Here's how the part is built. I have some questions about the finished solid (model axes, mm). A direction names the side the tool comes from. Coordinates: 2 decimals unless noted, no trailing zeros. Order: outer loops, then holes, each group sorted by start corner. A loop starts at its lowest first (then second) coordinate and runs counter-clockwise, first axis right, second up. Notation, with made-up numbers: (18, 78) - (64, 78) arc R23 cw to (64, 105) - close; hole circle Ø4 at (-7.5, 39.5). An arc over 180 degrees is marked (long way). Use one line per item in the form item = value. Start each with the question number.
from build123d import *

# Parameters (mm, degrees)
SKETCH_1_W          = 33
SKETCH_1_H          = 27
EXTRUDE_1_DEPTH     = 5
FILLET_1_R          = 2
SKETCH_2_R          = 1
EXTRUDE_2_DEPTH     = 8
SKETCH_3_W          = 10
SKETCH_3_H          = 10
EXTRUDE_3_DEPTH     = 6
CHAMFER_1_SIZE      = 1
CUT_EXTRUDE_1_DEPTH = 4
SKETCH_5_W          = 14.5
SKETCH_5_H          = 9
SKETCH_5_W_2        = 2.4
SKETCH_5_H_2        = 7.7
EXTRUDE_4_DEPTH     = 11
SKETCH_6_R          = 2.85
SKETCH_6_R_2        = 0.5
CUT_EXTRUDE_2_DEPTH = 8
CUT_EXTRUDE_2_DRAFT = -3
CUT_EXTRUDE_3_DEPTH = 11
EXTRUDE_5_DEPTH     = 7.5
SKETCH_9_W          = 7
SKETCH_9_H          = 4
EXTRUDE_6_DEPTH     = 4.3
FILLET_2_R          = 1
CUT_EXTRUDE_START   = -3.5
SKETCH_10_R         = 1.5
CUT_EXTRUDE_4_DEPTH = 2.5


with BuildPart() as part:
    # 草图1 → 凸台-拉伸1 (new body)
    with BuildSketch(Plane.XY):
        with Locations((16.5, 13.5)):
            Rectangle(SKETCH_1_W, SKETCH_1_H)
    extrude(amount=EXTRUDE_1_DEPTH)

    # 圆角1
    fillet_1_edges = [part.edges().sort_by_distance(p)[0] for p in [
        (33, 27, 2.5),
        (33, 0, 2.5),
    ]]
    fillet(fillet_1_edges, radius=FILLET_1_R)

    # 草图2 → 凸台-拉伸2 (add)
    with BuildSketch(Plane(origin=(0, 0, 0), x_dir=(-1, 0, 0), z_dir=(0, 0, -1))):
        with Locations((-17.2, 23.2)):
            Circle(SKETCH_2_R)
        with Locations((-29.5, 23.2)):
            Circle(SKETCH_2_R)
        with Locations((-29.5, 3.8)):
            Circle(SKETCH_2_R)
        with Locations((-17.2, 3.8)):
            Circle(SKETCH_2_R)
    extrude(amount=EXTRUDE_2_DEPTH)

    # 草图3 → 凸台-拉伸3 (add)
    with BuildSketch(Plane.XY.offset(5)):
        with Locations((28, 13.5)):
            Rectangle(SKETCH_3_W, SKETCH_3_H)
    extrude(amount=EXTRUDE_3_DEPTH)

    # 倒角1
    chamfer_1_edges = [part.edges().sort_by_distance(p)[0] for p in [
        (23, 8.5, 8),
    ]]
    chamfer(chamfer_1_edges, length=CHAMFER_1_SIZE)

    # 草图4 → 切除-拉伸1 (cut)
    with BuildSketch(Plane.XY.offset(11)):
        Polygon((24, 17.5), (27, 17.5), (27, 9.5), (25, 9.5), (24, 10.5), align=None)
        Polygon((29, 17.5), (32, 17.5), (32, 9.5), (30, 9.5), (29, 10.5), align=None)
    extrude(amount=-CUT_EXTRUDE_1_DEPTH, mode=Mode.SUBTRACT)

    # 草图5 → 凸台-拉伸4 (add)
    with BuildSketch(Plane.XY.offset(5)):
        with Locations((7.25, 20.5)):
            Rectangle(SKETCH_5_W, SKETCH_5_H)
        with Locations((9.8, 4.35)):
            Rectangle(SKETCH_5_W_2, SKETCH_5_H_2)
    extrude(amount=EXTRUDE_4_DEPTH)


with BuildPart() as cut_extrude_2_tool:
    # 草图6 → 切除-拉伸2 (with draft: the straight prism first)
    with BuildSketch(Plane.ZY):
        with Locations((11.55, 20.5)):
            Circle(SKETCH_6_R)
        with Locations((11.55, 20.5)):
            Circle(SKETCH_6_R_2, mode=Mode.SUBTRACT)
    extrude(amount=-CUT_EXTRUDE_2_DEPTH)
    # 切除-拉伸2: the draft: its side faces are tilted about the plane it starts from
    cut_extrude_2_sides = [cut_extrude_2_tool.faces().sort_by_distance(p)[0] for p in [
        (4, 20.5, 8.7),
        (4, 20.5, 11.05),
    ]]
    draft(cut_extrude_2_sides, Plane.ZY, CUT_EXTRUDE_2_DRAFT)


with BuildPart() as part_1:
    add(part.part)

    # 切除-拉伸2: cut by cut_extrude_2_tool
    add(cut_extrude_2_tool.part, mode=Mode.SUBTRACT)

    # 草图7 → 切除-拉伸3 (cut)
    with BuildSketch(Plane(origin=(14.5, 0, 0), x_dir=(0, 0, -1), z_dir=(1, 0, 0))):
        Polygon((-14.5, 18), (-14.5, 23), (-12.5, 25), (-16, 25), (-16, 16), (-12.5, 16), align=None)
    extrude(amount=-CUT_EXTRUDE_3_DEPTH, mode=Mode.SUBTRACT)

    # 草图8 → 凸台-拉伸5 (add)
    with BuildSketch(Plane.ZY):
        with BuildLine():
            Line((8.1, 9.95), (8.1, 4.15))
            ThreePointArc((8.1, 4.15), (6.55, 2.6), (5, 4.15))
            Line((5, 4.15), (5, 9.95))
            ThreePointArc((5, 9.95), (6.55, 11.5), (8.1, 9.95))
        make_face()
        with BuildLine():
            Line((7.6, 9.95), (7.6, 4.15))
            ThreePointArc((7.6, 4.15), (6.55, 3.1), (5.5, 4.15))
            Line((5.5, 4.15), (5.5, 9.95))
            ThreePointArc((5.5, 9.95), (6.55, 11), (7.6, 9.95))
        make_face(mode=Mode.SUBTRACT)
    extrude(amount=-EXTRUDE_5_DEPTH)

    # 草图9 → 凸台-拉伸6 (add)
    with BuildSketch(Plane.XY.offset(5)):
        with Locations((23, 24.5)):
            Rectangle(SKETCH_9_W, SKETCH_9_H)
        with Locations((23, 2.5)):
            Rectangle(SKETCH_9_W, SKETCH_9_H)
    extrude(amount=EXTRUDE_6_DEPTH)

    # 圆角2
    fillet_2_edges = [part_1.edges().sort_by_distance(p)[0] for p in [
        (1.75, 16, 16),
        (8.6, 4.35, 16),
        (9.8, 0.5, 16),
        (11, 4.35, 16),
        (9.8, 8.2, 16),
        (1.75, 25, 16),
        (0, 27, 2.5),
        (0, 0, 2.5),
    ]]
    fillet(fillet_2_edges, radius=FILLET_2_R)

    # 草图10 → 切除-拉伸4 (cut)
    with BuildSketch(Plane(origin=(0, 0, 0), x_dir=(-1, 0, 0), z_dir=(0, 0, -1)).offset(CUT_EXTRUDE_START)):
        with BuildLine():
            ThreePointArc((-33, 2), (-32.414213562, 0.585786438), (-31, 0))
            Line((-31, 0), (-1, 0))
            ThreePointArc((-1, 0), (-0.292893219, 0.292893219), (0, 1))
            Line((0, 1), (0, 26))
            ThreePointArc((0, 26), (-0.292893219, 26.707106781), (-1, 27))
            Line((-1, 27), (-31, 27))
            ThreePointArc((-31, 27), (-32.414213562, 26.414213562), (-33, 25))
            Line((-33, 25), (-33, 2))
        make_face()
        with Locations((-17.2, 3.8)):
            Circle(SKETCH_10_R, mode=Mode.SUBTRACT)
        with Locations((-29.5, 3.8)):
            Circle(SKETCH_10_R, mode=Mode.SUBTRACT)
        with Locations((-17.2, 23.2)):
            Circle(SKETCH_10_R, mode=Mode.SUBTRACT)
        with Locations((-29.5, 23.2)):
            Circle(SKETCH_10_R, mode=Mode.SUBTRACT)
    extrude(amount=CUT_EXTRUDE_4_DEPTH, mode=Mode.SUBTRACT)


solid = part_1.part
1) Suppose I cut it at C-C, the plane x = 4. List the corners of the cut face in (y, z) for me, then the cut area to 3 significant figures.
2) I need wall thicknesses on probe 1 along Y at (x, z) = (5, 6.5); probe 2 along Z at (x, y) = (25.5, 16.5); probe 3 along X at (y, z) = (17.5, 6). Which ranges of each line are inside material? Lowest first, please. Write a range as [from, to].
3) Suppose I cut it at A-A, the plane x = 23.5. List the corners of the cut face in (y, z) for me, then the cut area to 3 significant figures.
4) For pin 1 (2 mm diameter, centred on x = 7.5, y = 5.5, fed in from +Z); pin 2 (8 mm diameter, centred on x = 24.5, z = 12, fed in from -Y); pin 3 (5 mm diameter, centred on x = 30.5, z = 8.5, fed in from +Y), each with a flat end and sliding along its axis, tell me the tip position at first contact or that it passes through.
5) If we mould it in two halves opening along Y, with no side actions, what happens to faces 1 (the flat face through (0, 13.3, 0.5)), 2 (the cylindrical face through (32.4, 0.57, 4.26)), 3 (the cylindrical face through (30.61, 24.21, 2.27))? For each: pulls with the +Y half, pulls with the -Y half, needs draft (parallel to the pull), parting line crosses it, or undercut.
6) Suppose I cut it at B-B, the plane z = 11.55. List the corners of the cut face in (x, y) for me.
7) Which directions (+Z, -Z, +X, -X, +Y, -Y) give clear straight access to the entire face, cutting with the end or side of a thin tool? Please do faces 4 (the flat face through (10, 0.5, 10)), 5 (the flat face through (8.6, 4, 10)), 6 (the flat face through (9.1, 17, 13.5)), 7 (the flat face through (23, 25, 9.3)), 8 (the flat face through (23, 3, 9.3)).
From the geometry:
q1.outline = (0, 0) - (27, 0) - (27, 1) - (0, 1) - close; (0, 3.5) - (27, 3.5) - (27, 5) - (25, 5) - (25, 12.5) - (23, 14.5) - (18, 14.5) - (16, 12.5) - (16, 5) - (9.95, 5) arc R1.55 ccw to (9.95, 8.1) - (4.15, 8.1) arc R1.55 ccw to (4.15, 5) - (0, 5) - close; circle Ø1.42 at (20.5, 11.55); hole (4.15, 5.5) - (9.95, 5.5) arc R1.05 ccw to (9.95, 7.6) - (4.15, 7.6) arc R1.05 ccw to start; hole circle Ø5.28 at (20.5, 11.55)
q1.area = 139 mm2
q2.probe_1 = [2.6, 3.1], [11, 11.5], [16, 25]
q2.probe_2 = [0, 1], [3.5, 7]
q2.probe_3 = [0, 14.5], [23, 33]
q3.outline = (0, 0) - (27, 0) - (27, 1) - (0, 1) - close; (0, 3.5) - (27, 3.5) - (27, 5) - (26.5, 5) - (26.5, 9.3) - (22.5, 9.3) - (22.5, 5) - (18.5, 5) - (18.5, 11) - (9, 11) - (9, 5) - (4.5, 5) - (4.5, 9.3) - (0.5, 9.3) - (0.5, 5) - (0, 5) - close
q3.area = 159 mm2
q4.pin_1 = 8.1
q4.pin_2 = 0.5
q4.pin_3 = 18.5
q5.face_1 = needs draft
q5.face_2 = pulls with the -Y half
q5.face_3 = undercut
q6.outline = (0, 16) - (14.5, 16) - (14.5, 25) - (0, 25) - (0, 23.35) - (8, 22.93) - (8, 21.42) - (0, 21) - (0, 20) - (8, 19.58) - (8, 18.07) - (0, 17.65) - close; (8.6, 0.5) - (11, 0.5) - (11, 8.2) - (8.6, 8.2) - close
q7.face_4 = +Z, +X, -X, -Y
q7.face_5 = +Z, -Y
q7.face_6 = +Z, +X
q7.face_7 = +Z, +X, +Y
q7.face_8 = +Z, +X, -Y
